Model file for the job. Use its own axes, mm. A direction names the side the tool comes from. Round coordinates to 2 decimals unless told otherwise and drop trailing zeros. Loops run counter-clockwise (first coordinate to the right, second up) from the corner with the lowest first, then second, coordinate; pieces in that order, holes last. Notation, with made-up numbers: (39.25, -11) -> (80.25, -11) arc R22 cw to (80.25, 9) -> close; hole circle Ø11 at (26.5, 85). An arc over 180 degrees is marked (long way). Use a Markdown table: item, result.
from build123d import *

# Parameters (mm, degrees)
BOSS_EXTRUDE1_DEPTH = 3.81
BOSS_EXTRUDE2_START = 3.81
BOSS_EXTRUDE2_DEPTH = 11.43
SKETCH3_R           = 5.08
CUT_EXTRUDE1_DEPTH  = 20
SKETCH4_R           = 2.4892
CUT_EXTRUDE2_DEPTH  = 20


with BuildPart() as part:
    # Sketch1 → Boss-Extrude1 (new, symmetric)
    with BuildSketch(Plane.XY):
        with BuildLine():
            Line((-14.2875, 0), (14.2875, 0))
            Line((14.2875, 0), (12.692423957, 46.158604709))
            ThreePointArc((12.692423957, 46.158604709), (0, 58.42), (-12.692423957, 46.158604709))
            Line((-12.692423957, 46.158604709), (-14.2875, 0))
        make_face()
    extrude(amount=BOSS_EXTRUDE1_DEPTH, both=True)

    # Sketch2 → Boss-Extrude2 (add)
    with BuildSketch(Plane.XY.offset(BOSS_EXTRUDE2_START)):
        Polygon((-14.2875, 0), (14.2875, 0), (14.024180094, 7.62), (-14.024180094, 7.62), align=None)
    extrude(amount=BOSS_EXTRUDE2_DEPTH)

    # Sketch3 → Cut-Extrude1 (cut, symmetric)
    with BuildSketch(Plane.XY):
        with Locations((0, 45.72)):
            Circle(SKETCH3_R)
    extrude(amount=CUT_EXTRUDE1_DEPTH, both=True, mode=Mode.SUBTRACT)

    # Sketch4 → Cut-Extrude2 (cut, symmetric)
    with BuildSketch(Plane(origin=(0, 0, 0), x_dir=(1, 0, 0), z_dir=(0, 1, 0))):
        with Locations(Location((0, -9.525, 0), (0, 0, 270))):
            Circle(SKETCH4_R)
    extrude(amount=CUT_EXTRUDE2_DEPTH, both=True, mode=Mode.SUBTRACT)


solid = part.part
Q1. Band-saw the part on A-A, the plane x = 0. Give the cut face in (y, z), plus the area to 3 significant figures.
Results list:
| item | result |
|---|---|
| outline | (0, -3.81) -> (40.64, -3.81) -> (40.64, 3.81) -> (7.62, 3.81) -> (7.62, 7.04) -> (0, 7.04) -> close; (0, 12.01) -> (7.62, 12.01) -> (7.62, 15.24) -> (0, 15.24) -> close; (50.8, -3.81) -> (58.42, -3.81) -> (58.42, 3.81) -> (50.8, 3.81) -> close |
| area | 417 mm² |
Q2. Flat gauge pins, fed straight in: pin 1 (3 mm diameter, centred on y = 17.5, z = 4.5, fed in from -X); pin 2 (2 mm diameter, centred on x = -0.5, y = 19.5, fed in from +Z); pin 3 (1 mm diameter, centred on x = -9.5, z = 4, fed in from -Y). Where does each tip first touch, or does it go through?
Results list:
| item | result |
|---|---|
| pin 1 | stops at x = -13.73 |
| pin 2 | stops at z = 3.81 |
| pin 3 | stops at y = 0 |
Q3. Tool access for faces 1 (the face through (0, 4, 15.24)), 2 (the face through (3, 7.62, 9)): list every direction of +Z, -Z, +X, -X, +Y, -Y with a clear straight run to the whole face (end or side of a thin tool).
Results list:
| item | result |
|---|---|
| face 1 | +Z, +X, -X, +Y, -Y |
| face 2 | +Z, +X, -X, +Y |
Q4. Pull direction X, two halves, no side cores. Call faces 3 (the face through (0, 33, 3.81)), 4 (the face through (0.273, 58.417, 0.053)), 5 (the face through (0.75, 3.86, 11.9)): released by +X, released by -X, zero draft, split by the parting line, or undercut.
Results list:
| item | result |
|---|---|
| face 3 | zero draft |
| face 4 | split by the parting line |
| face 5 | undercut |
Q5. Band-saw the part on B-B, the plane z = -1.75. Give the cut face in (x, y), plus the area to 3 significant figures.
Results list:
| item | result |
|---|---|
| outline | (-14.29, 0) -> (14.29, 0) -> (12.69, 46.16) arc R12.7 ccw to (-12.69, 46.16) -> close; hole circle Ø10.16 at (0, 45.72) |
| area | 1,410 mm² |
Q6. Band-saw the part on C-C, the plane y = 25.5. Give the cut face in (x, z).
Results list:
| item | result |
|---|---|
| outline | (-13.41, -3.81) -> (13.41, -3.81) -> (13.41, 3.81) -> (-13.41, 3.81) -> close |
Q7. Drill centre lines: L1, parallel to Y at x = 0, z = 0.25; L2, parallel to Z at x = 9.5, y = 26; L3, parallel to Y at x = 7.25, z = 10.75. Where is each one in solid material? Low to high. Write a range as from..to.
Results list:
| item | result |
|---|---|
| L1 | y = 0..40.64, 50.8..58.42 |
| L2 | z = -3.81..3.81 |
| L3 | y = 0..7.62 |
Q8. Band-saw the part on D-D, the plane x = 10.5. Give the cut face in (y, z), plus the area to 3 significant figures.
Results list:
| item | result |
|---|---|
| outline | (0, -3.81) -> (52.86, -3.81) -> (52.86, 3.81) -> (7.62, 3.81) -> (7.62, 15.24) -> (0, 15.24) -> close |
| area | 490 mm² |
